from build123d import *


with BuildPart() as f1:
    # F0 (on Top) → F1 (revolve)
    with BuildSketch(Plane.XY):
        Polygon((0, 0), (0, 54), (-8, 54), (-8, 49.2), (-6, 49.2), (-6, 44.6), (-8, 44.6), (-8, 4.767014), (-4, 0), align=None)
    revolve(axis=Axis((0, 27, 0), (0, 1, 0)))


solid = f1.part
Can you work these out from the model? Positions are in its coordinate system, mm. A direction names the side the tool comes from. Give positions to 0.01 mm unless a question says otherwise; leave off trailing zeros. Loops run counter-clockwise (first coordinate to the right, second up) from the corner with the lowest first, then second, coordinate; pieces in that order, holes last. Notation, with made-up numbers: (7.25, 15.25) -> (39.25, 15.25) arc R13 ccw to (39.25, 33.25) -> close; hole circle Ø5 at (27.25, 84.25). An arc over 180 degrees is marked (long way). Use one line per item in the form item = value.
1) If we section it at A-A (z = 0): Please give me the cut outline in (x, y), plus the area to 3 significant figures.
Answers:
outline = (-8, 4.77) -> (-4, 0) -> (4, 0) -> (8, 4.77) -> (8, 44.6) -> (6, 44.6) -> (6, 49.2) -> (8, 49.2) -> (8, 54) -> (-8, 54) -> (-8, 49.2) -> (-6, 49.2) -> (-6, 44.6) -> (-8, 44.6) -> close
area = 827 mm²
2) If we section it at B-B (x = 0): Please give me the cut outline in (y, z).
Answers:
outline = (0, -4) -> (4.77, -8) -> (44.6, -8) -> (44.6, -6) -> (49.2, -6) -> (49.2, -8) -> (54, -8) -> (54, 8) -> (49.2, 8) -> (49.2, 6) -> (44.6, 6) -> (44.6, 8) -> (4.77, 8) -> (0, 4) -> close
3) I need wall thicknesses on line 1 along Y through (x, z) = (4.25, 6); line 2 along Y through (x, z) = (-6.75, 2); line 3 along Z through (x, y) = (-0.75, 21). Which ranges of each line are inside material? Lowest first, please.
Answers:
line_1 = 4 to 44.6, 49.2 to 54
line_2 = 3.62 to 44.6, 49.2 to 54
line_3 = -7.96 to 7.96
4) For faces 1 (the face through (-2, 44.6, 6)), 2 (the face through (-4, 0.23, 1.26)), which set-ups out of +Z, -Z, +X, -X, +Y, -Y let a thin tool reach every point of the face, with its end or its side?
Answers:
face_1 = none
face_2 = -Y
5) Will these pins go through, and if not, where does the flat tip stop? pin 1 (2 mm diameter, centred on y = 8.5, z = 1.5, fed in from +X); pin 2 (1 mm diameter, centred on x = -5.5, y = 27, fed in from +Z) (3 decimals); pin 3 (1.5 mm diameter, centred on x = 3.5, z = 4.5, fed in from -Y).
Answers:
pin_1 = 7.98
pin_2 = 6.245
pin_3 = 1.13
6) We'd pull the mould along Y, two halves only. Please class faces 3 (the face through (0, 0, 0)), 4 (the face through (1.73, 24.4, -7.81)), 5 (the face through (6, 47, 0)): released by +Y, released by -Y, zero draft, split by the parting line, or undercut.
Answers:
face_3 = released by -Y
face_4 = zero draft
face_5 = undercut
7) If we section it at D-D (y = 48.5): Please give me the cut outline in (x, z), plus the area to 3 significant figures.
Answers:
outline = circle Ø12 at (0, 0)
area = 113 mm²
8) If we section it at C-C (y = 14.5): Please give me the cut outline in (x, z), plus the area to 3 significant figures.
Answers:
outline = circle Ø16 at (0, 0)
area = 201 mm²
